Model file for the job. Use its own axes, mm. A direction names the side the tool comes from. Coordinates: 2 decimals unless noted, no trailing zeros. Write each loop counter-clockwise with the first axis right and the second up, starting at its lowest first coordinate (ties: lowest second). Pieces come first, ordered by that corner, then holes.
Q1. Band-saw the part on C-C, the plane y = 30. Write the cut outline in (x, z), plus the area to 3 significant figures.
Q2. Pull direction Y, two halves, no side cores. Call faces 1 (the flat face through (37.04, 2.43, 1.48)), 2 (the cylindrical face through (16.524, -8.979, 7.632)), 3 (the cylindrical face through (7.003, 8.641, -4.479)), 4 (the flat face through (5.8, 17, -4)): released by +Y, released by -Y, zero draft, split by the parting line, or undercut.
Q3. Pin check, flat tips, straight feed: P1, Ø1.5, axis at x = 12.5, z = 2, coming from the +Y side; P2, Ø1, axis at x = 26.5, z = -1.5, coming from the +Y side; P3, Ø3.5, axis at x = 18.5, y = 30, coming from the +Z side; P4, Ø16.5, axis at x = -14.5, y = -3.5, coming from the +Z side. Stop position of each tip, or through.
Q4. Which spindle directions (+Z, -Z, +X, -X, +Y, -Y) get a long thin tool onto all of the face, cutting with end or side? Do faces 5 (the cylindrical face through (6.941, 25.047, -4.479)), 6 (the flat face through (22.25, 30, -4)), 7 (the flat face through (-22.25, 30, -4)), 8 (the flat face through (-1, 9, -3)), 9 (the cylindrical face through (-21.537, 27.002, -4.479)). Say none if no direction does.
Q5. Drill centre lines: probe 1 along X at (y, z) = (-8.15, 7); probe 2 along Y at (x, z) = (-18.5, -3.7); probe 3 along Z at (x, y) = (24, -4). Where is each one in solid material? Low to high.
Q6. Band-saw the part on D-D, the plane z = 1.5. Write the cut outline in (x, y), plus the area to 3 significant figures.
Q7. Band-saw the part on A-A, the plane y = -1. Write the cut outline in (x, z), plus the area to 3 significant figures.
Q8. Band-saw the part on B-B, the plane x = 15. Write the cut outline in (y, z), plus the area to 3 significant figures.
from build123d import *

# Parameters (mm, degrees)
BOSS_EXTRUDE1_DEPTH = 3
SKETCH3_R           = 1.6
BOSS_EXTRUDE2_DEPTH = 3
SKETCH2_W           = 80
SKETCH2_H           = 3
BOSS_EXTRUDE3_DEPTH = 3
SKETCH8_W           = 80
SKETCH8_H           = 3
BOSS_EXTRUDE6_DEPTH = 16
SKETCH21_R          = 1.65
CUT_EXTRUDE1_DEPTH  = 4
CUT_EXTRUDE2_DEPTH  = 4


with BuildPart() as part:
    # Sketch1 → Boss-Extrude1 (new body)
    with BuildSketch(Plane.XY):
        Polygon((40, -2.5), (34, 7.5), (-34, 7.5), (-40, -2.5), (-40, -7.5), (40, -7.5), align=None)
    extrude(amount=BOSS_EXTRUDE1_DEPTH)



with BuildPart() as body_2:
    # Sketch3 → Boss-Extrude2 (new body)
    with BuildSketch(Plane(origin=(0, 0, -3), x_dir=(-1, 0, 0), z_dir=(0, 0, -1))):
        with BuildLine():
            Line((40, -7.5), (-40, -7.5))
            Line((-40, -7.5), (-40, -2.5))
            Line((-40, -2.5), (-34, 7.5))
            Line((-34, 7.5), (-9.8, 7.5))
            ThreePointArc((-9.8, 7.5), (-6.971572875, 8.671572875), (-5.8, 11.5))
            Line((-5.8, 11.5), (-5.8, 22.25))
            ThreePointArc((-5.8, 22.25), (-6.971572875, 25.078427125), (-9.8, 26.25))
            Line((-9.8, 26.25), (-19.75, 26.25))
            ThreePointArc((-19.75, 26.25), (-21.517766953, 26.982233047), (-22.25, 28.75))
            Line((-22.25, 28.75), (-22.25, 31.25))
            ThreePointArc((-22.25, 31.25), (-21.517766953, 33.017766953), (-19.75, 33.75))
            Line((-19.75, 33.75), (19.75, 33.75))
            ThreePointArc((19.75, 33.75), (21.517766953, 33.017766953), (22.25, 31.25))
            Line((22.25, 31.25), (22.25, 28.75))
            ThreePointArc((22.25, 28.75), (21.517766953, 26.982233047), (19.75, 26.25))
            Line((19.75, 26.25), (9.8, 26.25))
            ThreePointArc((9.8, 26.25), (6.971572875, 25.078427125), (5.8, 22.25))
            Line((5.8, 22.25), (5.8, 11.5))
            ThreePointArc((5.8, 11.5), (6.971572875, 8.671572875), (9.8, 7.5))
            Line((9.8, 7.5), (34, 7.5))
            Line((34, 7.5), (40, -2.5))
            Line((40, -2.5), (40, -7.5))
        make_face()
        with Locations((-18.5, 30)):
            Circle(SKETCH3_R, mode=Mode.SUBTRACT)
        with Locations((18.5, 30)):
            Circle(SKETCH3_R, mode=Mode.SUBTRACT)
    extrude(amount=BOSS_EXTRUDE2_DEPTH)


with BuildPart() as part_1:
    add(part.part)

    add(body_2.part)  # Boss-Extrude3 merges body 2
    # Sketch2 → Boss-Extrude3 (add)
    with BuildSketch(Plane(origin=(0, -7.5, 0), x_dir=(1, 0, 0), z_dir=(0, 1, 0))):
        with Locations((0, 4.5)):
            Rectangle(SKETCH2_W, SKETCH2_H)
        with Locations((0, 1.5)):
            Rectangle(SKETCH2_W, SKETCH2_H)
        with Locations((0, -1.5)):
            Rectangle(SKETCH2_W, SKETCH2_H)
    extrude(amount=-BOSS_EXTRUDE3_DEPTH)

    # Sketch8 → Boss-Extrude6 (add)
    with BuildSketch(Plane.XY.offset(3)):
        with Locations((0, -9)):
            Rectangle(SKETCH8_W, SKETCH8_H)
    extrude(amount=BOSS_EXTRUDE6_DEPTH)

    # Sketch21 → Cut-Extrude1 (cut, through all)
    with BuildSketch(Plane(origin=(0, -7.5, 0), x_dir=(1, 0, 0), z_dir=(0, 1, 0))):
        with Locations((-15, -7)):
            Circle(SKETCH21_R)
        with Locations((15, -7)):
            Circle(SKETCH21_R)
    extrude(amount=-CUT_EXTRUDE1_DEPTH, mode=Mode.SUBTRACT)

    # Sketch24 → Cut-Extrude2 (cut, through all)
    with BuildSketch(Plane(origin=(0, -7.5, 0), x_dir=(1, 0, 0), z_dir=(0, 1, 0))):
        Polygon((-40, -19), (-40, -9), (-34, -19), align=None)
        Polygon((40, -19), (34, -19), (40, -11), align=None)
    extrude(amount=-CUT_EXTRUDE2_DEPTH, mode=Mode.SUBTRACT)


solid = part_1.part
Answer sheet:
1. outline: (-22.25, -6) - (-20.1, -6) - (-20.1, -3) - (-22.25, -3) - close; (-16.9, -6) - (16.9, -6) - (16.9, -3) - (-16.9, -3) - close; (20.1, -6) - (22.25, -6) - (22.25, -3) - (20.1, -3) - close
1. area: 114 mm2
2. face 1: released by +Y
2. face 2: zero draft
2. face 3: undercut
2. face 4: undercut
3. P1: stops at y = 7.5
3. P2: stops at y = -7.5
3. P3: stops at z = -3
3. P4: stops at z = 19
4. face 5: +Z, -Z, +X
4. face 6: +Z, -Z, +X, +Y
4. face 7: +Z, -Z, -X, +Y
4. face 8: +X, -X, +Y
4. face 9: +Z, -Z, -X
5. probe 1: x = -40 to -16.65, -13.35 to 13.35, 16.65 to 40
5. probe 2: y = -10.5 to 7.5, 26.25 to 28.4, 31.6 to 33.75
5. probe 3: z = -6 to -3, 0 to 3
6. outline: (-40, -10.5) - (40, -10.5) - (40, -2.5) - (34, 7.5) - (-34, 7.5) - (-40, -2.5) - close
6. area: 1,380 mm2
7. outline: (-39.1, -6) - (39.1, -6) - (39.1, -3) - (-39.1, -3) - close; (-39.1, 0) - (39.1, 0) - (39.1, 3) - (-39.1, 3) - close
7. area: 469 mm2
8. outline: (-10.5, -6) - (7.5, -6) - (7.5, -3) - (-7.5, -3) - (-7.5, 0) - (7.5, 0) - (7.5, 3) - (-7.5, 3) - (-7.5, 5.35) - (-10.5, 5.35) - close; (-10.5, 8.65) - (-7.5, 8.65) - (-7.5, 19) - (-10.5, 19) - close; (26.25, -6) - (33.75, -6) - (33.75, -3) - (26.25, -3) - close
8. area: 178 mm2
